The listing builds one solid part. Answer for the finished solid, in the listing's coordinates (mm). Coordinates: 2 decimals unless noted, no trailing zeros. Order: outer loops, then holes, each group sorted by start corner. A loop starts at its lowest first (then second) coordinate and runs counter-clockwise, first axis right, second up. Notation, with made-up numbers: (-1, 33.5) -> (43, 33.5) arc R20 cw to (43, 71.5) -> close; hole circle Ø11 at (55, 81.25). An arc over 180 degrees is marked (long way). Return JSON: item names as keys, results as strings.
```python
from build123d import *

# Parameters (mm, degrees)
ESTRUSIONE_ESTRUSIONE1_DEPTH      = 10
ESTRUSIONE_ESTRUSIONE1_DEPTH_BACK = 10
SCHIZZO3_OUTSIDE_W                = 27.366
SCHIZZO3_OUTSIDE_H                = 13.749
TAGLIO_ESTRUSIONE2_DEPTH          = 9.355
TAGLIO_ESTRUSIONE2_DEPTH_BACK     = 9.355


with BuildPart() as part:
    # Schizzo2 → Estrusione-Estrusione1 (new body, two sides)
    with BuildSketch(Plane(origin=(0, 0, 0), x_dir=(0, 0, -1), z_dir=(1, 0, 0))) as estrusione_estrusione1_sk:
        Polygon((-7.200336343, -5.2), (7.199751527, -5.2), (8.355, 0), (8.355, 1.182571265), (-8.355, 1.182571265), (-8.355, 0), align=None)
    extrude(amount=ESTRUSIONE_ESTRUSIONE1_DEPTH)
    extrude(estrusione_estrusione1_sk.sketch, amount=-ESTRUSIONE_ESTRUSIONE1_DEPTH_BACK)

    # Schizzo3 outside → Taglio-Estrusione2 (cut, two sides)
    with BuildSketch(Plane.XY) as taglio_estrusione2_sk:
        with Locations((0, -2.0085)):
            Rectangle(SCHIZZO3_OUTSIDE_W, SCHIZZO3_OUTSIDE_H)
        Polygon((2.434296655, -5.201208291), (-2.434296655, -5.201208291), (-4.029664932, 0.001330674), (-4.029664932, 1.658816204), (4.029664932, 1.658816204), (4.029664932, 0.001330674), align=None, mode=Mode.SUBTRACT)
    extrude(amount=TAGLIO_ESTRUSIONE2_DEPTH, mode=Mode.SUBTRACT)
    extrude(taglio_estrusione2_sk.sketch, amount=-TAGLIO_ESTRUSIONE2_DEPTH_BACK, mode=Mode.SUBTRACT)


solid = part.part
```
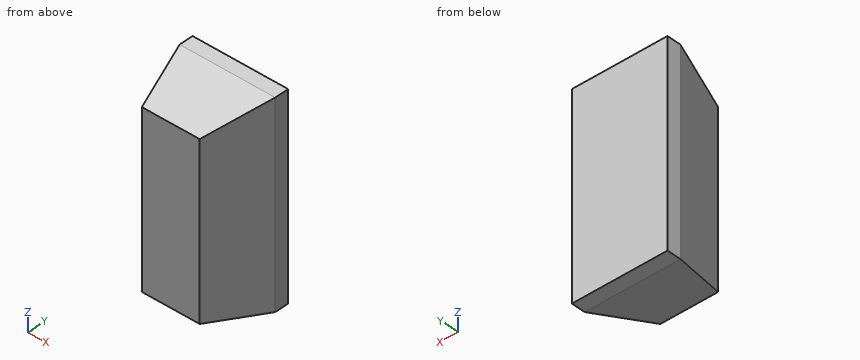
Item 1: Find the intervals of material crossed by probe 1 along Z at (x, y) = (-0.75, -0.5); probe 2 along X at (y, z) = (-4.5, -0.5); probe 3 along Z at (x, y) = (-0.25, -2.25), in increasing order.
Answer list:
{"probe 1": "-8.24 to 8.24", "probe 2": "-2.65 to 2.65", "probe 3": "-7.86 to 7.86"}
Item 2: The part is cut by section C-C on y = -3.5. Determine the outline of the cut face in (x, z).
Answer list:
{"outline": "(-2.96, -7.58) -> (2.96, -7.58) -> (2.96, 7.58) -> (-2.96, 7.58) -> close"}
Item 3: A flat-ended cylindrical pin translates along its axis: pin 1 (2 mm diameter, centred on y = -4.5, z = 0, fed in from +X). Find the tip coordinate at first contact, or state that the pin passes through.
Answer list:
{"pin 1": "x = 2.96"}
Item 4: The part is cut by section A-A on z = -2.5. Determine the outline of the cut face in (x, y).
Answer list:
{"outline": "(-4.03, 0) -> (-2.43, -5.2) -> (2.43, -5.2) -> (4.03, 0) -> (4.03, 1.18) -> (-4.03, 1.18) -> close"}
Item 5: The part is cut by section D-D on y = -0.25. Determine the outline of the cut face in (x, z).
Answer list:
{"outline": "(-3.95, -8.3) -> (3.95, -8.3) -> (3.95, 8.3) -> (-3.95, 8.3) -> close"}
Item 6: The part is cut by section B-B on x = -1.5. Determine the outline of the cut face in (y, z) (3 decimals), plus the area to 3 significant figures.
Answer list:
{"outline": "(-5.2, -7.2) -> (0, -8.355) -> (1.183, -8.355) -> (1.183, 8.355) -> (0, 8.355) -> (-5.2, 7.2) -> close", "area": "101 mm2"}
